Build history of the part. All positions in model axes, mm. A direction names the side the tool comes from. Give positions to 0.01 mm unless a question says otherwise; leave off trailing zeros. Order: outer loops, then holes, each group sorted by start corner. A loop starts at its lowest first (then second) coordinate and runs counter-clockwise, first axis right, second up. Notation, with made-up numbers: M 46.25,71.25 L 85.25,71.25 A12 ccw 85.25,83.25 Z; hole C 71.25,56.25 d8. An arc over 180 degrees is marked long. Use CSV: the item, a comma, the result in double quotes. Start each with the question number.
Item 1: Which spindle directions (+Z, -Z, +X, -X, +Y, -Y) get a long thin tool onto all of the face, cutting with end or side? Do faces 4 (the flat face through (6, 1, 14)), 5 (the flat face through (-6, 1, 14)), 6 (the flat face through (-3.15, 0.99, 16.45)), 7 (the cylindrical face through (-0.9, 8.44, -2.86)), 8 (the flat face through (0, 0, 1)). Say none if no direction does.
Item 2: Band-saw the part on B-B on z = 5.5. Write the cut outline in (x, y).
Item 3: Band-saw the part on A-A on y = 1. Write the cut outline in (x, z), plus the area to 3 significant figures.
Item 4: Pin check, flat tips, straight feed: P1, Ø5, axis at y = 6, z = 1.5, coming from the -X side; P2, Ø1.5, axis at y = 2, z = 7.5, coming from the +X side; P3, Ø2, axis at x = 1.5, y = 1, coming from the +Z side. Stop position of each tip, or through.
Item 5: Two-plate mould, pull along Z, no slides. Class faces 1 (the flat face through (-4, 1, 18.8)), 2 (the cylindrical face through (-0.631, 7.423, -2.003)), 3 (the flat face through (0, 2, 7)): pulls with the +Z half, pulls with the -Z half, needs draft (parallel to the pull), parting line crosses it, or undercut.
Item 6: Band-saw the part on C-C on x = -8.25. Write the cut outline in (y, z), plus the area to 3 significant figures.
Item 7: Band-saw the part on D-D on y = 5.75. Write the cut outline in (x, z).
Item 8: Wall check: line 1 along X through (y, z) = (1.3, 0); line 2 along X through (y, z) = (9, 0); line 3 along Y through (x, z) = (-3, 12.75). Give the ranges that are in metal, low to high.
from build123d import *

# Parameters (mm, degrees)
SKETCH1_R           = 0.25
BOSS_EXTRUDE1_DEPTH = 2
SKETCH2_R           = 10
SKETCH2_R_2         = 3
BOSS_EXTRUDE2_DEPTH = 2
SKETCH4_W           = 12
SKETCH4_H           = 0.2
CUT_EXTRUDE1_DEPTH  = 4
FILLET3_R           = 0.35
FILLET4_R           = 0.15
SKETCH5_R           = 3
SKETCH5_R_2         = 2.1
BOSS_EXTRUDE4_DEPTH = 13
FILLET5_R           = 2
FILLET6_R           = 2


with BuildPart() as part:
    # Sketch1 → Boss-Extrude1 (new body)
    with BuildSketch(Plane(origin=(0, 0, 0), x_dir=(1, 0, 0), z_dir=(0, 1, 0))):
        Polygon((-6, 6), (-6, -13.291502622), (-6, -19), (-2.70227506, -19), (-3.619175359, -13.8), (0, -13.8), (3.619175359, -13.8), (2.70227506, -19), (6, -19), (6, -13.291502622), (6, 6), align=None)
        with Locations(Location((0, 0, 0), (0, 0, 270))):
            Circle(SKETCH1_R, mode=Mode.SUBTRACT)
    extrude(amount=BOSS_EXTRUDE1_DEPTH)

    # Sketch2 → Boss-Extrude2 (add)
    with BuildSketch(Plane(origin=(0, 0, 0), x_dir=(1, 0, 0), z_dir=(0, 1, 0))):
        Circle(SKETCH2_R)
        Circle(SKETCH2_R_2, mode=Mode.SUBTRACT)
    extrude(amount=BOSS_EXTRUDE2_DEPTH)

    # Sketch4 → Cut-Extrude1 (cut)
    with BuildSketch(Plane(origin=(0, 2, 0), x_dir=(1, 0, 0), z_dir=(0, 1, 0))):
        with Locations((0, -18.9)):
            Rectangle(SKETCH4_W, SKETCH4_H)
    extrude(amount=-CUT_EXTRUDE1_DEPTH, mode=Mode.SUBTRACT)

    # Fillet3
    fillet3_edges = [part.edges().sort_by_distance(p)[0] for p in [
        (3.619175359, 1, 13.8),
        (-3.619175359, 1, 13.8),
    ]]
    fillet(fillet3_edges, radius=FILLET3_R)

    # Fillet4
    fillet4_edges = [part.edges().sort_by_distance(p)[0] for p in [
        (2.737540456, 1, 18.8),
        (-2.737540456, 1, 18.8),
    ]]
    fillet(fillet4_edges, radius=FILLET4_R)

    # Sketch5 → Boss-Extrude4 (add)
    with BuildSketch(Plane(origin=(0, 0, 0), x_dir=(1, 0, 0), z_dir=(0, 1, 0))):
        with Locations(Location((0, 0, 0), (0, 0, 90))):
            Circle(SKETCH5_R)
        with Locations(Location((0, 0, 0), (0, 0, 90))):
            Circle(SKETCH5_R_2, mode=Mode.SUBTRACT)
    extrude(amount=BOSS_EXTRUDE4_DEPTH)

    # Fillet5
    fillet5_edges = [part.edges().sort_by_distance(p)[0] for p in [
        (0, 2, 3),
    ]]
    fillet(fillet5_edges, radius=FILLET5_R)

    # Fillet6
    fillet6_edges = [part.edges().sort_by_distance(p)[0] for p in [
        (6, 1, 8),
        (-6, 1, 8),
    ]]
    fillet(fillet6_edges, radius=FILLET6_R)


solid = part.part
Model answer:
1,face 4,"+Z, +X, +Y, -Y"
1,face 5,"+Z, -X, +Y, -Y"
1,face 6,"+Y, -Y"
1,face 7,"+Y"
1,face 8,"+Z, -Z, +X, -X, -Y"
2,outline,"M -8.35,0 L 8.35,0 L 8.35,2 L -8.35,2 Z"
3,outline,"M -6.67,7.45 A10 ccw long 6.67,7.45 A2 cw 6,8.94 L 6,18.8 L 2.92,18.8 A0.15 ccw 2.77,18.62 L 3.55,14.21 A0.35 cw 3.2,13.8 L -3.2,13.8 A0.35 cw -3.55,14.21 L -2.77,18.62 A0.15 ccw -2.92,18.8 L -6,18.8 L -6,8.94 A2 cw Z; hole C 0,0 d0.5"
3,area,"396 mm^2"
4,P1,"stops at x = -3"
4,P2,"stops at x = 7.38"
4,P3,"stops at z = 13.8"
5,face 1,"pulls with the +Z half"
5,face 2,"undercut"
5,face 3,"needs draft"
6,outline,"M 0,-5.65 L 2,-5.65 L 2,5.65 L 0,5.65 Z"
6,area,"22.6 mm^2"
7,outline,"C 0,0 d6; hole C 0,0 d4.2"
8,line 1,"x = -10 to -0.25, 0.25 to 10"
8,line 2,"x = -3 to -2.1, 2.1 to 3"
8,line 3,"y = 0 to 2"
